```python
from build123d import *

# Parameters (mm, degrees)
REVOLU_O3_ANGLE                             = 10
CORTE_EXTRUS_O2_DEPTH                       = 10
BROCA_DE_ROSQUEAR_PARA_TARRAXA_DE_M41_D     = 3.3
BROCA_DE_ROSQUEAR_PARA_TARRAXA_DE_M41_DEPTH = 10
BROCA_DE_ROSQUEAR_PARA_TARRAXA_DE_M41_TIP   = 0.991420021
FILETE1_R                                   = 0.25


with BuildPart() as part:
    # Esboço1 → Revolução2 (revolve)
    with BuildSketch(Plane.XY, mode=Mode.PRIVATE) as revolu_o2_sk:
        Polygon((3.1, 5.6), (3.5, 0), (0, 0), (0, 5.6), align=None)
    revolve(revolu_o2_sk.sketch.rotate(Axis((0, 0, 0), (0, 1, 0)), 90), axis=Axis((0, 0, 0), (0, 1, 0)))

    # Esboço3 → Revolução3 (revolve)
    with BuildSketch(Plane.XY):
        with BuildLine():
            Line((3.1, 5.6), (3.159667096, 6.470663935))
            ThreePointArc((3.159667096, 6.470663935), (6.735500159, 8.547793041), (7.332110812, 4.455714945))
            Line((7.332110812, 4.455714945), (3.429154002, 0.895958371))
            Line((3.429154002, 0.895958371), (3.1, 5.6))
        make_face()
    revolve(axis=Axis((0, 0, 0), (0, 1, 0)), revolution_arc=REVOLU_O3_ANGLE)

    # Esboço4 → Corte-extrusão2 (cut)
    with BuildSketch(Plane(origin=(0, 5.6, 0), x_dir=(1, 0, 0), z_dir=(0, 1, 0))):
        with BuildLine():
            Line((0.270182803, -3.088203564), (0, 0))
            Line((0, 0), (-0.270182803, 3.088203564))
            ThreePointArc((-0.270182803, 3.088203564), (-3.088203564, -0.270182803), (0.270182803, -3.088203564))
        make_face()
        with BuildLine():
            Line((0.342968893, -3.920152382), (0.270182803, -3.088203564))
            ThreePointArc((0.270182803, -3.088203564), (-3.088203564, -0.270182803), (-0.270182803, 3.088203564))
            Line((-0.270182803, 3.088203564), (-0.342968893, 3.920152382))
            ThreePointArc((-0.342968893, 3.920152382), (-3.920152382, -0.342968893), (0.342968893, -3.920152382))
        make_face()
    extrude(amount=-CORTE_EXTRUS_O2_DEPTH, mode=Mode.SUBTRACT)

    # Espelhar1: part across face


with BuildPart() as part_1:
    add(part.part)
    add(part.part.mirror(Plane(origin=(0, 2.743434343, 0), x_dir=(0.08715574300604889, 0, 0.9961946980691392), z_dir=(-0.9961946980691393, 0, 0.08715574300604889))))

    # Broca de rosquear para tarraxa de M41
    with Locations(Plane(origin=(0, 5.6, 0), x_dir=(1, 0, 0), z_dir=(0, 1, 0))):
        with Locations((0, 0)):
            Hole(BROCA_DE_ROSQUEAR_PARA_TARRAXA_DE_M41_D / 2, depth=BROCA_DE_ROSQUEAR_PARA_TARRAXA_DE_M41_DEPTH)
            with Locations((0, 0, -(BROCA_DE_ROSQUEAR_PARA_TARRAXA_DE_M41_DEPTH + BROCA_DE_ROSQUEAR_PARA_TARRAXA_DE_M41_TIP / 2))):  # 118° drill point
                Cone(0, BROCA_DE_ROSQUEAR_PARA_TARRAXA_DE_M41_D / 2, BROCA_DE_ROSQUEAR_PARA_TARRAXA_DE_M41_TIP, mode=Mode.SUBTRACT)

    # Filete1
    # the kernel refuses this fillet: 0.25 mm, written as the material it takes off along each edge
    with BuildSketch(Plane(origin=(0, 5.6, 0), x_dir=(0.08715574274766005, 0, 0.9961946980917454), z_dir=(-0.9961946980917454, 0, 0.08715574274766005))) as filete1_piece_1:
        with BuildLine():
            CenterArc((3.1 - FILETE1_R * 0.931119203401, -FILETE1_R), FILETE1_R, 4.08561678, 85.91438322)
            Line((3.1 - FILETE1_R * 0.931119203401, 0), (3.1, 0))
            Line((3.1, 0), (3.1 + FILETE1_R * 0.0663394964294, -FILETE1_R * 0.928752950012))
        make_face()
    revolve(axis=Axis((0, 5.6, 0), (0, 1, 0)), revolution_arc=85, mode=Mode.SUBTRACT)
    with BuildSketch(Plane(origin=(0, 5.6, 0), x_dir=(0.08715574274766005, 0, 0.9961946980917454), z_dir=(-0.9961946980917454, 0, 0.08715574274766005))) as filete1_piece_2_section:
        with BuildLine():
            CenterArc((3.1 - FILETE1_R * 0.931119203401, -FILETE1_R), FILETE1_R, 4.08561678, 85.91438322)
            Line((3.1 - FILETE1_R * 0.931119203401, 0), (3.1, 0))
            Line((3.1, 0), (3.1 + FILETE1_R * 0.0663394964294, -FILETE1_R * 0.928752950012))
        make_face()
    filete1_piece_2 = revolve(axis=Axis((0, 5.6, 0), (0, 1, 0)), revolution_arc=95.759741079, mode=Mode.PRIVATE)
    filete1_piece_2 = split(filete1_piece_2, bisect_by=Plane(origin=(3.054670317, 5.486797578, -0.538620794), z_dir=(-0.17364817766693072, 0, -0.984807753012208)), keep=Keep.TOP, mode=Mode.PRIVATE)
    add(filete1_piece_2, mode=Mode.SUBTRACT)
    with BuildSketch(Plane(origin=(0, 0, 0), x_dir=(0.08715574274766182, 0, 0.9961946980917452), z_dir=(-0.9961946980917452, 0, 0.08715574274766182))) as filete1_piece_3:
        with BuildLine():
            CenterArc((3.5 - FILETE1_R * 1.07397634626, FILETE1_R), FILETE1_R, 270, 94.08561678)
            Line((3.5 - FILETE1_R * 1.07397634626, 0), (3.5, 0))
            Line((3.5, 0), (3.5 - FILETE1_R * 0.0765176464277, FILETE1_R * 1.07124704999))
        make_face()
    revolve(axis=Axis((0, 0, 0), (0, 1, 0)), revolution_arc=180, mode=Mode.SUBTRACT)
    with BuildSketch(Plane(origin=(0, 5.6, 0), x_dir=(-0.08715574274762866, 0, -0.9961946980917481), z_dir=(-0.9961946980917481, 0, 0.08715574274762866))) as filete1_piece_4:
        with BuildLine():
            CenterArc((3.1 - FILETE1_R * 0.931119203401, FILETE1_R), FILETE1_R, 270, 85.91438322)
            Line((3.1 - FILETE1_R * 0.931119203401, 0), (3.1, 0))
            Line((3.1, 0), (3.1 + FILETE1_R * 0.0663394964294, FILETE1_R * 0.928752950012))
        make_face()
    revolve(axis=Axis((0, 5.6, 0), (0, -1, 0)), revolution_arc=85, mode=Mode.SUBTRACT)
    with BuildSketch(Plane(origin=(0, 5.6, 0), x_dir=(-0.08715574274762866, 0, -0.9961946980917481), z_dir=(-0.9961946980917481, 0, 0.08715574274762866))) as filete1_piece_5_section:
        with BuildLine():
            CenterArc((3.1 - FILETE1_R * 0.931119203401, FILETE1_R), FILETE1_R, 270, 85.91438322)
            Line((3.1 - FILETE1_R * 0.931119203401, 0), (3.1, 0))
            Line((3.1, 0), (3.1 + FILETE1_R * 0.0663394964294, FILETE1_R * 0.928752950012))
        make_face()
    filete1_piece_5 = revolve(axis=Axis((0, 5.6, 0), (0, -1, 0)), revolution_arc=95.759741079, mode=Mode.PRIVATE)
    filete1_piece_5 = split(filete1_piece_5, bisect_by=Plane(origin=(3.10179353, 5.486797578, 0), z_dir=(0, 0, 1)), keep=Keep.TOP, mode=Mode.PRIVATE)
    add(filete1_piece_5, mode=Mode.SUBTRACT)
    with BuildSketch(Plane(origin=(0, 5.6, 0), x_dir=(-0.08715574326446912, 0, -0.9961946980465305), z_dir=(0.9961946980465305, 0, -0.08715574326446912))) as filete1_piece_6:
        with BuildLine():
            CenterArc((3.1 - FILETE1_R * 0.931119203401, -FILETE1_R), FILETE1_R, 4.08561678, 85.91438322)
            Line((3.1 + FILETE1_R * 0.0663394964294, -FILETE1_R * 0.928752950012), (3.1, 0))
            Line((3.1, 0), (3.1 - FILETE1_R * 0.931119203401, 0))
        make_face()
    revolve(axis=Axis((0, 5.6, 0), (0, 1, 0)), revolution_arc=85, mode=Mode.SUBTRACT)
    with BuildSketch(Plane(origin=(0, 5.6, 0), x_dir=(-0.08715574326446912, 0, -0.9961946980465305), z_dir=(0.9961946980465305, 0, -0.08715574326446912))) as filete1_piece_7_section:
        with BuildLine():
            CenterArc((3.1 - FILETE1_R * 0.931119203401, -FILETE1_R), FILETE1_R, 4.08561678, 85.91438322)
            Line((3.1 + FILETE1_R * 0.0663394964294, -FILETE1_R * 0.928752950012), (3.1, 0))
            Line((3.1, 0), (3.1 - FILETE1_R * 0.931119203401, 0))
        make_face()
    filete1_piece_7 = revolve(axis=Axis((0, 5.6, 0), (0, 1, 0)), revolution_arc=95.759741079, mode=Mode.PRIVATE)
    filete1_piece_7 = split(filete1_piece_7, bisect_by=Plane(origin=(-2.996372834, 5.561029125, 0.528341377), z_dir=(0.17364817817780473, 0, 0.9848077529221271)), keep=Keep.TOP, mode=Mode.PRIVATE)
    add(filete1_piece_7, mode=Mode.SUBTRACT)
    with BuildSketch(Plane(origin=(0, 0, 0), x_dir=(0.08715574326443595, 0, 0.9961946980465334), z_dir=(0.9961946980465334, 0, -0.08715574326443595))) as filete1_piece_8:
        with BuildLine():
            CenterArc((3.5 - FILETE1_R * 1.07397634626, -FILETE1_R), FILETE1_R, 355.91438322, 94.08561678)
            Line((3.5 - FILETE1_R * 1.07397634626, 0), (3.5, 0))
            Line((3.5, 0), (3.5 - FILETE1_R * 0.0765176464277, -FILETE1_R * 1.07124704999))
        make_face()
    revolve(axis=Axis((0, 0, 0), (0, -1, 0)), revolution_arc=180, mode=Mode.SUBTRACT)
    with BuildSketch(Plane(origin=(0, 5.6, 0), x_dir=(0.08715574326443776, 0, 0.996194698046533), z_dir=(0.996194698046533, 0, -0.08715574326443776))) as filete1_piece_9:
        with BuildLine():
            CenterArc((3.1 - FILETE1_R * 0.931119203401, FILETE1_R), FILETE1_R, 270, 85.91438322)
            Line((3.1 + FILETE1_R * 0.0663394964294, FILETE1_R * 0.928752950012), (3.1, 0))
            Line((3.1, 0), (3.1 - FILETE1_R * 0.931119203401, 0))
        make_face()
    revolve(axis=Axis((0, 5.6, 0), (0, -1, 0)), revolution_arc=85, mode=Mode.SUBTRACT)
    with BuildSketch(Plane(origin=(0, 5.6, 0), x_dir=(0.08715574326443776, 0, 0.996194698046533), z_dir=(0.996194698046533, 0, -0.08715574326443776))) as filete1_piece_10_section:
        with BuildLine():
            CenterArc((3.1 - FILETE1_R * 0.931119203401, FILETE1_R), FILETE1_R, 270, 85.91438322)
            Line((3.1 + FILETE1_R * 0.0663394964294, FILETE1_R * 0.928752950012), (3.1, 0))
            Line((3.1, 0), (3.1 - FILETE1_R * 0.931119203401, 0))
        make_face()
    filete1_piece_10 = revolve(axis=Axis((0, 5.6, 0), (0, -1, 0)), revolution_arc=95.759741079, mode=Mode.PRIVATE)
    filete1_piece_10 = split(filete1_piece_10, bisect_by=Plane(origin=(-3.042596715, 5.561029125, 2e-09), z_dir=(-5.187550944363294e-10, 0, -1.0)), keep=Keep.TOP, mode=Mode.PRIVATE)
    add(filete1_piece_10, mode=Mode.SUBTRACT)


solid = part_1.part
```
CAD build for the part. Positions are in the model's coordinates, mm. Round coordinates to 2 decimals unless told otherwise and drop trailing zeros. Loops run counter-clockwise (first coordinate to the right, second up) from the corner with the lowest first, then second, coordinate; pieces in that order, holes last. Notation, with made-up numbers: M -6.75,64.25 L -1.75,64.25 A27 cw -1.75,82.25 Z; hole C 84,-11 d6. An arc over 180 degrees is marked long. Return JSON: item names as keys, results as strings. Group by question number.
(1) Mould opens along X. For faces 1 (the conical face through (5.337, 2.654, -0.46)), 2 (the cylindrical face through (1.216, 2.761, -1.115)), 3 (the flat face through (-6, 6, 0)), 4 (the flat face through (-5.459, 5.781, 0.963)) say: +X half, -X half, draft (parallel to the pull), parting line (faces both ways), or undercut.
(2) Drop flat-ended pins along their axis: P1, Ø2.5, axis at x = -6, y = 5, coming from the -Z side; P2, Ø1.5, axis at y = 3.5, z = 2, coming from the +X side; P3, Ø2.5, axis at x = 5.5, y = 7, coming from the +Z side. Give the stop position or say it passes through.
(3) Saw through at C-C, the plane y = 4.75. List the corners of the cut face in (x, z).
(4) Wall check: probe 1 along Z at (x, y) = (0, 3.7); probe 2 along Y at (x, z) = (-2.5, 1.5); probe 3 along Z at (x, y) = (0, 2.1). Give the ranges that are in metal, low to high. Write a range as [from, to].
(5) Saw through at A-A, the plane y = 2.25. List the corners of the cut face in (x, z).
Answer list:
{
 "1": {"face 1": "+X half", "face 2": "undercut", "face 3": "draft", "face 4": "undercut"},
 "2": {"P1": "z = 0", "P2": "x = 3.01", "P3": "z = 0"},
 "3": {"outline": "M -7.61,0 L -3.16,0 A3.16 ccw 3.11,-0.55 L 7.49,-1.32 A7.61 ccw 7.61,0 L 3.16,0 A3.16 ccw -3.11,0.55 L -7.49,1.32 A7.61 ccw Z; hole C 0,0 d3.3"},
 "4": {"probe 1": "[-3.24, -1.65], [1.65, 3.24]", "probe 2": "[0, 5.6]", "probe 3": "[-3.35, -1.65], [1.65, 3.35]"},
 "5": {"outline": "M -4.91,0 L -3.34,0 A3.34 ccw 3.29,-0.58 L 4.84,-0.85 A4.91 ccw 4.91,0 L 3.34,0 A3.34 ccw -3.29,0.58 L -4.84,0.85 A4.91 ccw Z; hole C 0,0 d3.3"}
}
